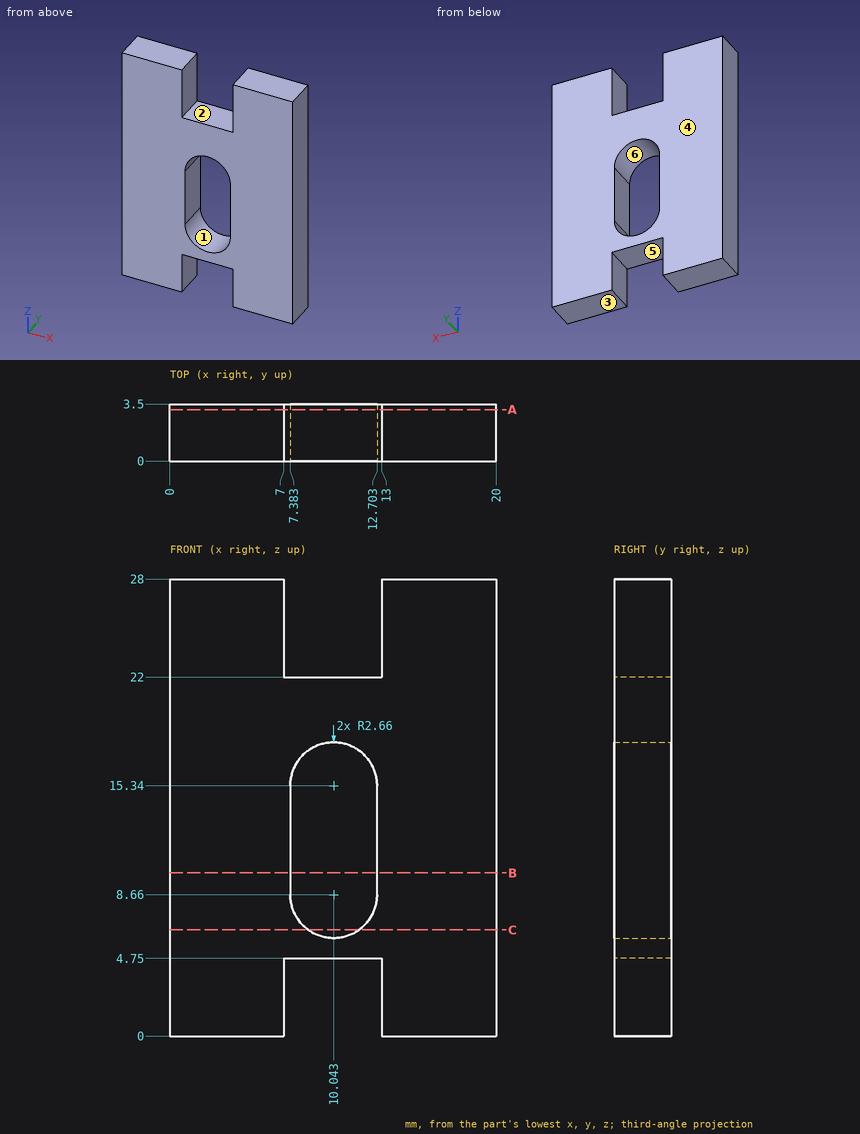
Geometry check sheet. Reference: drawing and pictorial views, mm from the part's lowest x, y, z. A direction names the side the tool comes from. Give positions to 0.01 mm unless a question says otherwise; leave off trailing zeros. Order: outer loops, then holes, each group sorted by start corner. A loop starts at its lowest first (then second) coordinate and runs counter-clockwise, first axis right, second up. Notation, with made-up numbers: M 85,25.25 L 120,25.25 A14 cw 120,32.25 Z; hole C 30.5,19.25 d8. An arc over 180 degrees is marked long. Use one line per item in the form item = value. Start each with the question number.
Q1. Section check B-B (z = 10). Enter the section's corners in (x, y).
Q2. Mould release check, pull along X, two halves, no side actions. Record for the marked faces 1, 2 and 3: +X half, -X half, draft (parallel to the pull), parting line (faces both ways), or undercut.
Q3. Scan lines: line 1 along X through (y, z) = (0.6, 8.5); line 2 along X through (y, z) = (2.95, 23); line 3 along Z through (x, y) = (10, 2.8). Record each from-to range of solid material in increasing order. Write a range as [from, to].
Q4. Section check C-C (z = 6.5). Enter the section's corners in (x, y).
Q5. Go/stop test with a flat-tipped pin: pin 1 Ø1.8 at (x, y) = (8.5, 2.5) entering from -Z. Record where the tip stops, or that it passes through.
Q6. Access from +Z, -Z, +X, -X, +Y, -Y to the whole of each face (thin tool, end or side, straight path). Record for the marked faces 4, 5 and 6.
Q7. Section check A-A (y = 3.15). Enter the section's corners in (x, z).
Evaluation:
q1.outline = M 0,0 L 7.38,0 L 7.38,3.5 L 0,3.5 Z; M 12.7,0 L 20,0 L 20,3.5 L 12.7,3.5 Z
q2.face_1 = undercut
q2.face_2 = undercut
q2.face_3 = draft
q3.line_1 = [0, 7.39], [12.7, 20]
q3.line_2 = [0, 7], [13, 20]
q3.line_3 = [4.75, 6], [18, 22]
q4.outline = M 0,0 L 8.49,0 L 8.49,3.5 L 0,3.5 Z; M 11.6,0 L 20,0 L 20,3.5 L 11.6,3.5 Z
q5.pin_1 = 4.75
q6.face_4 = +Z, -Z, +X, -X, +Y
q6.face_5 = -Z, +Y, -Y
q6.face_6 = +Y, -Y
q7.outline = M 0,0 L 7,0 L 7,4.75 L 13,4.75 L 13,0 L 20,0 L 20,28 L 13,28 L 13,22 L 7,22 L 7,28 L 0,28 Z; hole M 7.38,8.66 A2.66 ccw 12.7,8.66 L 12.7,15.34 A2.66 ccw 7.38,15.34 Z
